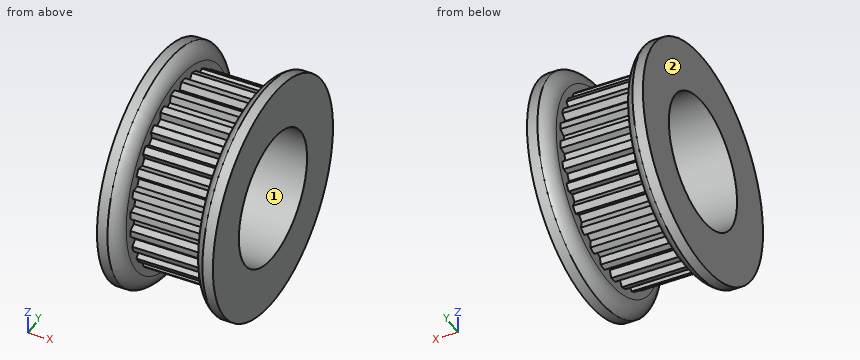
```python
from build123d import *

# Parameters (mm, degrees)
SKETCH4_R          = 9.0551
SKETCH4_R_2        = 8.89635
CUT_EXTRUDE2_DEPTH = 7.112
CUT_EXTRUDE1_DEPTH = 7.112
CIRPATTERN1_COUNT  = 28
SKETCH6_R          = 6.35
CUT_EXTRUDE3_DEPTH = 24.562439751
SPLIT1_START       = -8.7376
SPLIT1_OUTLINE_R   = 8.7376
SPLIT1_OUTLINE_R_2 = 6.35
SPLIT1_DEPTH       = 6.35


# Read off the part's stored shape, not the designer's step: Split1
with BuildPart() as part:
    # Sketch1 → Revolve1 (revolve)
    with BuildSketch(Plane.XY, mode=Mode.PRIVATE) as revolve1_sk:
        with BuildLine():
            Line((-8.7376, 3.175), (8.7376, 3.175))
            Line((8.7376, 3.175), (8.7376, 11.176))
            Line((8.7376, 11.176), (7.7343, 11.176))
            ThreePointArc((7.7343, 11.176), (7.003726949, 10.549537058), (6.731, 9.6266))
            Line((6.731, 9.6266), (6.731, 9.0551))
            Line((6.731, 9.0551), (-0.381, 9.0551))
            Line((-0.381, 9.0551), (-0.381, 9.6266))
            ThreePointArc((-0.381, 9.6266), (-0.653726949, 10.549537058), (-1.3843, 11.176))
            Line((-1.3843, 11.176), (-2.3876, 11.176))
            Line((-2.3876, 11.176), (-2.3876, 8.7376))
            Line((-2.3876, 8.7376), (-8.7376, 8.7376))
            Line((-8.7376, 8.7376), (-8.7376, 3.175))
        make_face()
    revolve(revolve1_sk.sketch.rotate(Axis((-8.7376, 0, 0), (1, 0, 0)), 90), axis=Axis((-8.7376, 0, 0), (1, 0, 0)))

    # Sketch4 → Cut-Extrude2 (cut)
    with BuildSketch(Plane(origin=(-0.381, 0, 0), x_dir=(0, 0, -1), z_dir=(1, 0, 0))):
        Circle(SKETCH4_R)
        Circle(SKETCH4_R_2, mode=Mode.SUBTRACT)
    extrude(amount=CUT_EXTRUDE2_DEPTH, mode=Mode.SUBTRACT)

    # Sketch3 → Cut-Extrude1 (cut)
    with BuildSketch(Plane(origin=(-0.381, 0, 0), x_dir=(0, 0, -1), z_dir=(1, 0, 0))):
        with BuildLine():
            Line((-0.643388094, 8.873054439), (-0.340062676, 8.222570981))
            Line((-0.340062676, 8.222570981), (0.340062676, 8.222570981))
            Line((0.340062676, 8.222570981), (0.643388094, 8.873054439))
            ThreePointArc((0.643388094, 8.873054439), (0, 8.89635), (-0.643388094, 8.873054439))
        make_face()
    cut_extrude1 = extrude(amount=CUT_EXTRUDE1_DEPTH, mode=Mode.SUBTRACT)

    # CirPattern1: Cut-Extrude1 ×28 about axis
    cirpattern1_axis = Axis((0, 0, 0), (1, 0, 0))
    for i in range(1, CIRPATTERN1_COUNT):
        add(cut_extrude1.rotate(cirpattern1_axis, i * 360 / CIRPATTERN1_COUNT), mode=Mode.SUBTRACT)

    # Sketch6 → Cut-Extrude3 (cut, through all)
    with BuildSketch(Plane.ZY.offset(8.7376)):
        Circle(SKETCH6_R)
    extrude(amount=-CUT_EXTRUDE3_DEPTH, mode=Mode.SUBTRACT)

    # Split1 outline → Split1 (cut)
    with BuildSketch(Plane.YZ.offset(SPLIT1_START)):
        Circle(SPLIT1_OUTLINE_R)
        Circle(SPLIT1_OUTLINE_R_2, mode=Mode.SUBTRACT)
    extrude(amount=SPLIT1_DEPTH, mode=Mode.SUBTRACT)


solid = part.part
```
Can you work these out from the model? Positions are in its coordinate system, mm. Face numbers are marked on the shaded views. Coordinates: 2 decimals unless noted, no trailing zeros. Order: outer loops, then holes, each group sorted by start corner. A loop starts at its lowest first (then second) coordinate and runs counter-clockwise, first axis right, second up.
1. If we section it at A-A (z = 0): Please give me the cut outline in (x, y), then the cut area to 3 significant figures.
2. Thinking about a two-plate mould opening in Y: for the marked faces 1 and 2, which applies, +Y half, -Y half, draft (parallel to the pull), parting line (faces both ways), or undercut?
3. I need wall thicknesses on line 1 (X direction, y = -0.25, z = -9); line 2 (Z direction, x = 5.5, y = 0). Which ranges of each line are inside material? Lowest first, please.
4. I'm going to push flat-ended pins straight in: pin 1 (6 mm diameter, centred on y = 0, z = -2, fed in from +X); pin 2 (6 mm diameter, centred on x = 1.5, y = 3.5, fed in from -Z); pin 3 (2 mm diameter, centred on x = 5.5, z = -6.5, fed in from +Y); pin 4 (4 mm diameter, centred on x = 5.5, z = 6, fed in from -Y). Where does each tip first touch, or does it pass through?
Entries:
1. outline: (-2.39, -11.18) - (-1.38, -11.18) arc R1.7 ccw to (-0.38, -9.63) - (-0.38, -8.22) - (6.73, -8.22) - (6.73, -9.63) arc R1.7 ccw to (7.73, -11.18) - (8.74, -11.18) - (8.74, -6.35) - (-2.39, -6.35) - close; (-2.39, 6.35) - (8.74, 6.35) - (8.74, 11.18) - (7.73, 11.18) arc R1.7 ccw to (6.73, 9.63) - (6.73, 8.22) - (-0.38, 8.22) - (-0.38, 9.63) arc R1.7 ccw to (-1.38, 11.18) - (-2.39, 11.18) - close
1. area: 63.6 mm2
2. face 1: undercut
2. face 2: draft
3. line 1: x = -2.39 to -0.38, 6.73 to 8.74
3. line 2: z = -8.22 to -6.35, 6.35 to 8.22
4. pin 1: passes through
4. pin 2: stops at z = -10.87
4. pin 3: stops at y = 6.54
4. pin 4: stops at y = -9.61
